Autodesk Inventor part; units mm, degrees
ref_plane "YZ Plane" through (0, 0, 0) normal (1, 0, 0) x (0, 1, 0)
ref_plane "XZ Plane" through (0, 0, 0) normal (0, 1, 0) x (-1, 0, 0)
ref_plane "XY Plane" through (0, 0, 0) normal (0, 0, 1) x (1, 0, 0)
sketch "Szkic1" plane through (0, 0, 0) normal (0, 1, 0) x (-1, 0, 0)
  line L0 (-13.25, 25) -> (19.25, 25)
  line L1 (19.25, 25) -> (19.25, -25)
  line L2 (19.25, -25) -> (-13.25, -25)
  line L3 (-19.25, 25) -> (19.25, -25) construction
  line L4 (19.25, 25) -> (-19.25, -25) construction
  line L5 (19.25, 0) -> (38.5, 0) construction
  line L6 (19.25, 0) -> (0.25, 0)
  line L7 (19.25, 0) -> (38.25, 0) construction
  circle A0 centre (0.25, 0) radius 8
  line L8 (19.25, 25) -> (-13.25, 25)
  line L9 (19.25, 25) -> (51.75, 25) construction
  arc A1 (-19.25, 0) -> (-13.25, -13.9642) centre (0, 0) ccw
  arc A2 (-13.25, 13.9642) -> (-19.25, 0) centre (0, 0) ccw
  line L10 (-13.25, 25) -> (-13.25, 13.9642)
  line L11 (-13.25, -13.9642) -> (-13.25, -25)
  point P0 (0, 0)
  dimension "d1" = 50
  dimension "d4" = 19
  dimension "d5" = 180
  dimension "d6" = 16
  dimension "d7" = 32.5
  dimension "d8" = 180
extrude "Wyciągnięcie proste1" add sketch "Szkic1" along normal blind 85
sketch "Szkic2" plane through (0, 0, 0) normal (0, -1, 0) x (1, 0, 0)
  circle A0 centre (-0.25, 0) radius 8
  circle A1 centre (-0.25, 0) radius 9.5
  circle A2 centre (-0.25, 0) radius 17
  circle A3 centre (-0.25, 0) radius 15.5
  point P0 (0, 0)
  dimension "d11" = 19
  dimension "d12" = 34
  dimension "d13" = 31
extrude "Wyciągnięcie proste2" cut sketch "Szkic2" against normal blind 1
sketch "Szkic3" plane through (-0.25, 0, 0) normal (0, -1, 0) x (1, 0, 0)
  circle A0 centre (0, 0) radius 9.5
  circle A1 centre (0, 0) radius 15.5
  point P0 (0.25, 0)
extrude "Wyciągnięcie proste3" cut sketch "Szkic3" against normal blind 2
sketch "Szkic4" plane through (0, 85, 0) normal (0, 1, 0) x (1, 0, 0)
  circle A0 centre (-0.25, 0) radius 8
  circle A1 centre (-0.25, 0) radius 9.5
  circle A2 centre (-0.25, 0) radius 17
  circle A3 centre (-0.25, 0) radius 15.5
  point P0 (0, 0)
  point P1 (0, 0)
  dimension "d18" = 19
  dimension "d19" = 34
  dimension "d20" = 31
extrude "Wyciągnięcie proste4" cut sketch "Szkic4" against normal blind 1
sketch "Szkic5" plane through (-0.25, 85, 0) normal (0, 1, 0) x (1, 0, 0)
  circle A0 centre (0, 0) radius 9.5
  circle A1 centre (0, 0) radius 15.5
  point P0 (0.25, 0)
extrude "Wyciągnięcie proste5" cut sketch "Szkic5" against normal blind 2
properties part number "Łożysko liniowe w obudowie SMAG16UU-L"
Read the model definition and answer for the solid it produces. Units are mm, in the model's axes. A direction names the side the tool comes from. Give positions to 0.01 mm unless a question says otherwise; leave off trailing zeros. Write each loop counter-clockwise with the first axis right and the second up, starting at its lowest first coordinate (ties: lowest second). Pieces come first, ordered by that corner, then holes. Notation, with made-up numbers: (54, -36.5) - (61, -36.5) arc R21 ccw to (61, -11.5) - close; hole circle Ø4 at (13, 60). An arc over 180 degrees is marked (long way). Answer in a Markdown table with one row per item. Add a question column.
Item 1: Section D-D, the plane z = -21.5 is taken. Write down the section's boundary in (x, y), and give its area (3 significant figures).
Item 2: Find the intervals of material crossed by L1, parallel to X at y = 83.4, z = 0; L2, parallel to Z at x = -0.25, y = 83.6; L3, parallel to Z at x = -0.25, y = 84.6, in increasing order.
Item 3: Determine the mould class of faces 1 (the face through (-3, 42, 25)), 2 (the face through (-4, 85, 17)), 3 (the face through (4.13, 83.51, 8.43)), 4 (the face through (17.643, 41.905, -7.7)) for opening direction Z: pulls with the +Z half, pulls with the -Z half, needs draft (parallel to the pull), parting line crosses it, or undercut.
Item 4: Section B-B, the plane y = 33.5 is taken. Write down the section's boundary in (x, z).
Item 5: Flat-ended cylindrical pins translate along their axes: P1, Ø6, axis at y = 31.5, z = 9.5, coming from the +X side; P2, Ø10, axis at x = -8.5, z = -5, coming from the -Y side; P3, Ø21, axis at x = 0, z = 0.5, coming from the +Y side. Find the tip coordinate at first contact, or state that the pin passes through.
Item 6: A tool of negligible diameter and unlimited length cuts with its end or side. For faces 5 (the face through (1.48, 41.92, 7.81)), 6 (the face through (4.13, 1.49, -8.43)), 7 (the face through (-2.268, 83.507, -15.368)), 8 (the face through (13.25, 42, -19)), from which of +Z, -Z, +X, -X, +Y, -Y can it reach the whole face along a straight path? Write none if from no direction.
Recorded:
| question | item | result |
|---|---|---|
| 1 | outline | (-19.25, 0) - (13.25, 0) - (13.25, 85) - (-19.25, 85) - close |
| 1 | area | 2,760 mm2 |
| 2 | L1 | x = -19.25 to -15.75, -9.75 to -8.25, 7.75 to 9.25, 15.25 to 19.25 |
| 2 | L2 | z = -25 to -15.5, -9.5 to -8, 8 to 9.5, 15.5 to 25 |
| 2 | L3 | z = -25 to -17, 17 to 25 |
| 3 | face 1 | pulls with the +Z half |
| 3 | face 2 | needs draft |
| 3 | face 3 | undercut |
| 3 | face 4 | pulls with the -Z half |
| 4 | outline | (-19.25, -25) - (13.25, -25) - (13.25, -13.96) arc R19.25 ccw to (19.25, 0) arc R19.25 ccw to (13.25, 13.96) - (13.25, 25) - (-19.25, 25) - close; hole circle Ø16 at (-0.25, 0) |
| 5 | P1 | stops at x = 18.12 |
| 5 | P2 | stops at y = 1 |
| 5 | P3 | stops at y = 84 |
| 6 | face 5 | +Y, -Y |
| 6 | face 6 | -Y |
| 6 | face 7 | +Y |
| 6 | face 8 | -Z, +X, +Y, -Y |
